Work out the finished part from the listing and answer in its coordinate system (mm). Face numbers are marked on the shaded views. Coordinates: 2 decimals unless noted, no trailing zeros. Order: outer loops, then holes, each group sorted by start corner. A loop starts at its lowest first (then second) coordinate and runs counter-clockwise, first axis right, second up. Notation, with made-up numbers: M 80,30.25 L 113,30.25 A24 cw 113,53.25 Z; hole C 64.25,76.5 d7. An arc over 180 degrees is marked long. Use a Markdown table: item, result.
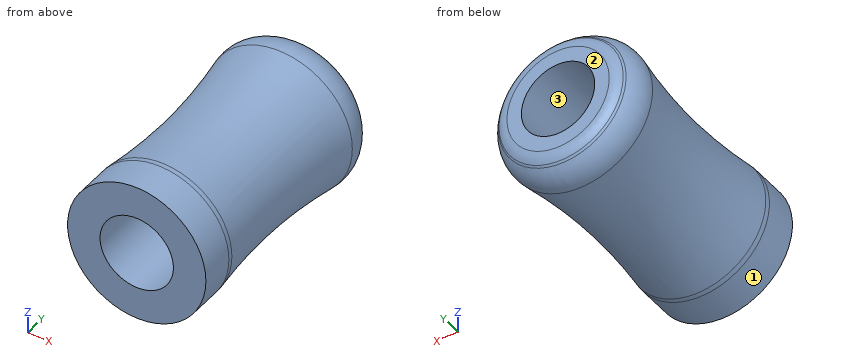
from build123d import *

# Parameters (mm, degrees)
F2_R     = 2
F3_R     = 9.75
F3_R_2   = 8.95
F4_DEPTH = 10
F5_R     = 5


with BuildPart() as f1:
    # F0 (on Top) → F1 (revolve)
    with BuildSketch(Plane.XY):
        with BuildLine():
            ThreePointArc((9.75, -15), (8.281654, -1.025091), (9.37742, 12.983957))
            ThreePointArc((9.37742, 12.983957), (9.246485, 14.870996), (8.263125, 16.486875))
            Line((8.263125, 16.486875), (7.45, 17.3))
            Line((7.45, 17.3), (4.75, 17.3))
            Line((4.75, 17.3), (4.75, -15))
            Line((4.75, -15), (9.75, -15))
        make_face()
    revolve(axis=Axis((0, -4.586624, 0), (0, -1, 0)))

    # F2
    f2_edges = [f1.edges().sort_by_distance(p)[0] for p in [
        (-7.45, 17.3, 0),
    ]]
    fillet(f2_edges, radius=F2_R)

    # F3 (on face) → F4 (cut)
    with BuildSketch(Plane.XZ.offset(15)):
        Circle(F3_R)
        Circle(F3_R_2, mode=Mode.SUBTRACT)
    extrude(amount=-F4_DEPTH, mode=Mode.SUBTRACT)

    # F5
    f5_edges = [f1.edges().sort_by_distance(p)[0] for p in [
        (-8.95, -10.174491, 0),
        (8.287942, 1.420896, 0),
        (-9.37742, 12.983957, 0),
    ]]
    fillet(f5_edges, radius=F5_R)


solid = f1.part
(1) A cutting plane is placed at A-A (y = 8). Determine the outline of the cut face in (x, z).
Conclusion:
| item | result |
|---|---|
| outline | C 0,0 d17.38; hole C 0,0 d9.5 |
(2) Determine the mould class of the marked faces 1, 2 and 3 for opening direction Z: pulls with the +Z half, pulls with the -Z half, needs draft (parallel to the pull), parting line crosses it, or undercut.
Conclusion:
| item | result |
|---|---|
| face 1 | parting line crosses it |
| face 2 | needs draft |
| face 3 | undercut |
(3) Given P1, Ø3, axis at x = -5.5, y = 9.5, coming from the -Z side; P2, Ø5, axis at y = 14, z = -5, coming from the -X side; P3, Ø6, axis at y = -8.5, z = -6, coming from the -X side, each flat-ended and moving along its own axis, determine where each tip first touches the part or whether it passes through.
Conclusion:
| item | result |
|---|---|
| P1 | z = -7.94 |
| P2 | x = -9.09 |
| P3 | x = -8.28 |
(4) Straight lines are drawn through the part: L1, parallel to Z at x = 0, y = -6.5; L2, parallel to X at y = 1, z = 0.75; L3, parallel to X at y = 6, z = -1. For each, find the intervals that lie inside material, in ascending order.
Conclusion:
| item | result |
|---|---|
| L1 | -8.55 to -4.75, 4.75 to 8.55 |
| L2 | -8.25 to -4.69, 4.69 to 8.25 |
| L3 | -8.45 to -4.64, 4.64 to 8.45 |
(5) A cutting plane is placed at B-B (y = 2.5). Determine the outline of the cut face in (x, z).
Conclusion:
| item | result |
|---|---|
| outline | C 0,0 d16.63; hole C 0,0 d9.5 |
